Input: part model. Units: mm. Frame: model coordinates. Face numbers are marked on the shaded views. A direction names the side the tool comes from. Coordinates: 2 decimals unless noted, no trailing zeros. Order: outer loops, then holes, each group sorted by start corner. A loop starts at its lowest first (then second) coordinate and runs counter-clockwise, first axis right, second up. Notation, with made-up numbers: (71, -13) -> (121, -13) arc R14 cw to (121, 8) -> close; hole circle Ø5 at (78, 66.25). An arc over 180 degrees is marked (long way). Write each question's results on one line, items separated by ' | '.
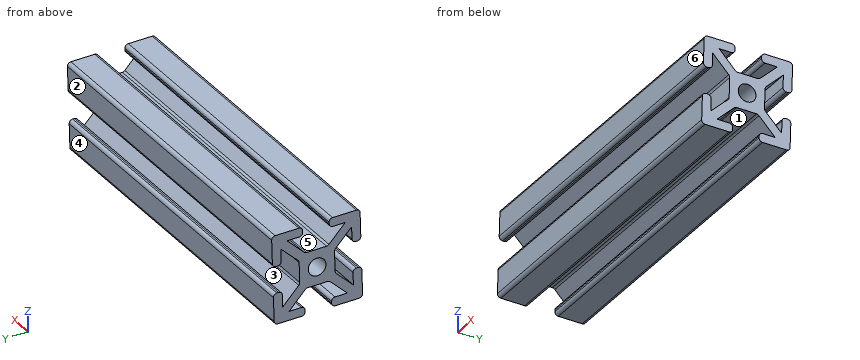
```python
from build123d import *

# Parameters (mm, degrees)
SKETCH11_R       = 2
SIZE_4X4_1_DEPTH = 80


with BuildPart() as part:
    # Sketch11 → Size 4X4 (1) (new body)
    with BuildSketch(Plane(origin=(0, 0, 0), x_dir=(-0.05317143033370503, 0, -0.9985853989500688), z_dir=(0.9985853989500688, 0, -0.05317143033370503))):
        with BuildLine():
            Line((-3, 9.2), (-3, 8.8))
            ThreePointArc((-3, 8.8), (-3.234314575, 8.234314575), (-3.8, 8))
            Line((-3.8, 8), (-6.585786438, 8))
            Line((-6.585786438, 8), (-2.820101013, 4.234314575))
            ThreePointArc((-2.820101013, 4.234314575), (-2.560562334, 4.060896374), (-2.254415588, 4))
            Line((-2.254415588, 4), (2.254415588, 4))
            ThreePointArc((2.254415588, 4), (2.560562334, 4.060896374), (2.820101013, 4.234314575))
            Line((2.820101013, 4.234314575), (6.585786438, 8))
            Line((6.585786438, 8), (3.8, 8))
            ThreePointArc((3.8, 8), (3.234314575, 8.234314575), (3, 8.8))
            Line((3, 8.8), (3, 9.2))
            ThreePointArc((3, 9.2), (3.234314575, 9.765685425), (3.8, 10))
            Line((3.8, 10), (9.2, 10))
            ThreePointArc((9.2, 10), (9.765685425, 9.765685425), (10, 9.2))
            Line((10, 9.2), (10, 3.8))
            ThreePointArc((10, 3.8), (9.765685425, 3.234314575), (9.2, 3))
            Line((9.2, 3), (8.8, 3))
            ThreePointArc((8.8, 3), (8.234314575, 3.234314575), (8, 3.8))
            Line((8, 3.8), (8, 6.585786438))
            Line((8, 6.585786438), (4.234314575, 2.820101013))
            ThreePointArc((4.234314575, 2.820101013), (4.060896374, 2.560562334), (4, 2.254415588))
            Line((4, 2.254415588), (4, -2.254415588))
            ThreePointArc((4, -2.254415588), (4.060896374, -2.560562334), (4.234314575, -2.820101013))
            Line((4.234314575, -2.820101013), (8, -6.585786438))
            Line((8, -6.585786438), (8, -3.8))
            ThreePointArc((8, -3.8), (8.234314575, -3.234314575), (8.8, -3))
            Line((8.8, -3), (9.2, -3))
            ThreePointArc((9.2, -3), (9.765685425, -3.234314575), (10, -3.8))
            Line((10, -3.8), (10, -9.2))
            ThreePointArc((10, -9.2), (9.765685425, -9.765685425), (9.2, -10))
            Line((9.2, -10), (3.8, -10))
            ThreePointArc((3.8, -10), (3.234314575, -9.765685425), (3, -9.2))
            Line((3, -9.2), (3, -8.8))
            ThreePointArc((3, -8.8), (3.234314575, -8.234314575), (3.8, -8))
            Line((3.8, -8), (6.585786438, -8))
            Line((6.585786438, -8), (2.820101013, -4.234314575))
            ThreePointArc((2.820101013, -4.234314575), (2.560562334, -4.060896374), (2.254415588, -4))
            Line((2.254415588, -4), (-2.254415588, -4))
            ThreePointArc((-2.254415588, -4), (-2.560562334, -4.060896374), (-2.820101013, -4.234314575))
            Line((-2.820101013, -4.234314575), (-6.585786438, -8))
            Line((-6.585786438, -8), (-3.8, -8))
            ThreePointArc((-3.8, -8), (-3.234314575, -8.234314575), (-3, -8.8))
            Line((-3, -8.8), (-3, -9.2))
            ThreePointArc((-3, -9.2), (-3.234314575, -9.765685425), (-3.8, -10))
            Line((-3.8, -10), (-9.2, -10))
            ThreePointArc((-9.2, -10), (-9.765685425, -9.765685425), (-10, -9.2))
            Line((-10, -9.2), (-10, -3.8))
            ThreePointArc((-10, -3.8), (-9.765685425, -3.234314575), (-9.2, -3))
            Line((-9.2, -3), (-8.8, -3))
            ThreePointArc((-8.8, -3), (-8.234314575, -3.234314575), (-8, -3.8))
            Line((-8, -3.8), (-8, -6.585786438))
            Line((-8, -6.585786438), (-4.234314575, -2.820101013))
            ThreePointArc((-4.234314575, -2.820101013), (-4.060896374, -2.560562334), (-4, -2.254415588))
            Line((-4, -2.254415588), (-4, 2.254415588))
            ThreePointArc((-4, 2.254415588), (-4.060896374, 2.560562334), (-4.234314575, 2.820101013))
            Line((-4.234314575, 2.820101013), (-8, 6.585786438))
            Line((-8, 6.585786438), (-8, 3.8))
            ThreePointArc((-8, 3.8), (-8.234314575, 3.234314575), (-8.8, 3))
            Line((-8.8, 3), (-9.2, 3))
            ThreePointArc((-9.2, 3), (-9.765685425, 3.234314575), (-10, 3.8))
            Line((-10, 3.8), (-10, 9.2))
            ThreePointArc((-10, 9.2), (-9.765685425, 9.765685425), (-9.2, 10))
            Line((-9.2, 10), (-3.8, 10))
            ThreePointArc((-3.8, 10), (-3.234314575, 9.765685425), (-3, 9.2))
        make_face()
        Circle(SKETCH11_R, mode=Mode.SUBTRACT)
    extrude(amount=SIZE_4X4_1_DEPTH)


solid = part.part
```
(1) Pin query (flat end, axial travel): P1, Ø6, axis at y = 3, z = -0.5, coming from the -X side; P2, Ø5.5, axis at x = 21, z = 1.5, coming from the +Y side; P3, Ø6, axis at y = 4.5, z = 4, coming from the -X side; P4, Ø2, axis at y = 0.5, z = -8, coming from the +X side. Return the tip coordinate at first contact, or that it passes through.
Return value:
P1: x = -0.19 | P2: y = 10 | P3: x = 0.06 | P4: x = 79.74
(2) Mould query, pull axis Y, two halves, no side actions, for the marked faces 4, 5 and 6. Classes: +Y half, -Y half, draft (parallel to the pull), parting line (faces both ways), or undercut.
Return value:
face 4: +Y half | face 5: undercut | face 6: -Y half
(3) Reachability of the marked faces 1, 2 and 3 from +Z, -Z, +X, -X, +Y, -Y: full face, straight path, thin tool, end or side. Return the list, or none.
Return value:
face 1: -Z, -X | face 2: +Z, -Z, +X, -X, +Y | face 3: +X
(4) Line query: line 1 along Z through (x, y) = (43.5, -4.25); line 2 along Y through (x, z) = (76.5, 1.75); line 3 along Z through (x, y) = (68, -3.75). Output: solid intervals per line, ascending. Write a range as from..to.
Return value:
line 1: -12.33..-10.33, -7.99..-5.16, 0.52..3.36, 5.7..7.7 | line 2: -10..-8, -7.23..-4.4, 4.4..7.23, 8..10 | line 3: -13.63..-11.63, -8.79..1.55, 4.39..6.39
(5) Cut plane A-A, the plane y = 5.5. Return loops of the section in (x, z), plus the area to 3 significant figures.
Return value:
outline: (-0.53, -9.99) -> (79.36, -14.24) -> (79.46, -12.24) -> (-0.43, -7.99) -> close; (-0.37, -6.9) -> (79.52, -11.16) -> (79.67, -8.33) -> (-0.22, -4.08) -> close; (0.22, 4.08) -> (80.1, -0.17) -> (80.25, 2.65) -> (0.37, 6.9) -> close; (0.43, 7.99) -> (80.31, 3.73) -> (80.42, 5.73) -> (0.53, 9.99) -> close | area: 773 mm2
